Could you check a few things on this model? Use its own coordinates, in mm. A direction names the side the tool comes from. Give positions to 0.01 mm unless a question says otherwise; leave off trailing zeros. Loops run counter-clockwise (first coordinate to the right, second up) from the corner with the lowest first, then second, coordinate; pieces in that order, holes last. Notation, with made-up numbers: (0, 81.5) -> (34, 81.5) arc R28 cw to (34, 110.5) -> close; hole circle Ø4 at (63.25, 44). An arc over 180 degrees is marked (long way). Write item = value, one per line. Start each with the question number.
1) I want a section at A-A (x = -1.25). List the corners of the cut face in (y, z) for me.
2) I want a section at D-D (z = 7.25). List the corners of the cut face in (x, y) for me (3 decimals), and give its area (3 significant figures).
3) I want a section at C-C (z = 0.5). Count the separate pieces of the cut face and the enclosed holes in it, and give its area (3 significant figures).
4) If we mould it in two halves opening along Y, with no side actions, what happens to faces 1 (the face through (-10, -12, 10.9)), 2 (the face through (7.805, 8.803, 9.632)), 3 (the face through (12.93, 12.9, 7.54))? For each: +Y half, -Y half, draft (parallel to the pull), parting line (faces both ways), or undercut.
5) I need wall thicknesses on probe 1 along Y at (x, z) = (-10, 6) (3 decimals); probe 2 along X at (y, z) = (10, 7.5) (3 decimals). Which ranges of each line are inside material? Lowest first, please. Write a range as from..to.
6) On a 3-axis mill with a long thin cutter (end or side, diameter ignored), from which of +Z, -Z, +X, -X, +Y, -Y can I reach the whole of each face in a straight line? I mean faces 4 (the face through (7.824, 8.768, -1.232)), 5 (the face through (12.176, -11.232, 9.632)), 6 (the face through (9.46, -12.44, 4.16)), 7 (the face through (-11, -13.5, 1)). Say none if no direction works.
7) I want a section at B-B (y = 7). List the corners of the cut face in (x, z) for me, and give its area (3 significant figures).
8) I'm going to push flat-ended pins straight in: pin 1 Ø1.5 at (x, z) = (-9.5, 4) entering from +Y; pin 2 Ø4 at (x, y) = (-5, -9.5) entering from +Z; pin 3 Ø13.5 at (x, y) = (4.5, 0) entering from -Z. Where does each tip first touch, or does it pass through?
from build123d import *

# Parameters (mm, degrees)
F1_R      = 1.575
F2_DEPTH  = 1.7
F3_R      = 1.575
F4_DEPTH  = 2.5
F5_R      = 2.5
F5_R_2    = 1.575
F6_DEPTH  = 5
F7_R      = 1.575
F8_DEPTH  = 1.7
F9_R      = 1.575
F10_DEPTH = 2.5


with BuildPart() as f2:
    # F1 (on Top) → F2 (new body)
    with BuildSketch(Plane.XY):
        with BuildLine():
            Line((-10.2, 13.5), (-11.5, 13.5))
            ThreePointArc((-11.5, 13.5), (-12.9142135624, 12.9142135624), (-13.5, 11.5))
            Line((-13.5, 11.5), (-13.5, -11.5))
            ThreePointArc((-13.5, -11.5), (-12.9142135624, -12.9142135624), (-11.5, -13.5))
            Line((-11.5, -13.5), (-10.2, -13.5))
            Line((-10.2, -13.5), (10.2, -13.5))
            Line((10.2, -13.5), (11.5, -13.5))
            ThreePointArc((11.5, -13.5), (12.9142135624, -12.9142135624), (13.5, -11.5))
            Line((13.5, -11.5), (13.5, 11.5))
            ThreePointArc((13.5, 11.5), (12.9142135624, 12.9142135624), (11.5, 13.5))
            Line((11.5, 13.5), (10.2, 13.5))
            Line((10.2, 13.5), (-10.2, 13.5))
        make_face()
        with Locations((-10, -10)):
            Circle(F1_R, mode=Mode.SUBTRACT)
        with Locations((10, -10)):
            Circle(F1_R, mode=Mode.SUBTRACT)
        with Locations((-10, 10)):
            Circle(F1_R, mode=Mode.SUBTRACT)
        with Locations((10, 10)):
            Circle(F1_R, mode=Mode.SUBTRACT)
        with BuildLine():
            Line((-5.5434908481, 18.2035445979), (-10.2, 13.5))
            Line((-10.2, 13.5), (10.2, 13.5))
            Line((10.2, 13.5), (5.5434908481, 18.2035445979))
            ThreePointArc((5.5434908481, 18.2035445979), (5.2178432469, 18.4229151093), (4.832839739, 18.5))
            Line((4.832839739, 18.5), (-4.832839739, 18.5))
            ThreePointArc((-4.832839739, 18.5), (-5.2178432469, 18.4229151093), (-5.5434908481, 18.2035445979))
        make_face()
        with BuildLine():
            Line((10.2, -13.5), (-10.2, -13.5))
            Line((-10.2, -13.5), (-5.5434908481, -18.2035445979))
            ThreePointArc((-5.5434908481, -18.2035445979), (-5.2178432469, -18.4229151093), (-4.832839739, -18.5))
            Line((-4.832839739, -18.5), (4.832839739, -18.5))
            ThreePointArc((4.832839739, -18.5), (5.2178432469, -18.4229151093), (5.5434908481, -18.2035445979))
            Line((5.5434908481, -18.2035445979), (10.2, -13.5))
        make_face()
    extrude(amount=F2_DEPTH)

    # F3 (on face) → F4 (join)
    with BuildSketch(Plane(origin=(0, 0, 0), x_dir=(1, 0, 0), z_dir=(0, 0, -1))):
        Polygon((-11.4020402321, -7.4765863358), (-12.8863604535, -9.952495626), (-11.4843202214, -12.4759092903), (-8.5979597679, -12.5234136642), (-7.1136395465, -10.047504374), (-8.5156797786, -7.5240907097), align=None)
        with Locations((-10, -10)):
            Circle(F3_R, mode=Mode.SUBTRACT)
        Polygon((-12.8863604535, 9.952495626), (-11.4020402321, 7.4765863358), (-8.5156797786, 7.5240907097), (-7.1136395465, 10.047504374), (-8.5979597679, 12.5234136642), (-11.4843202214, 12.4759092903), align=None)
        with Locations((-10, 10)):
            Circle(F3_R, mode=Mode.SUBTRACT)
        Polygon((11.4843202214, -12.4759092903), (12.8863604535, -9.952495626), (11.4020402321, -7.4765863358), (8.5156797786, -7.5240907097), (7.1136395465, -10.047504374), (8.5979597679, -12.5234136642), align=None)
        with Locations((10, -10)):
            Circle(F3_R, mode=Mode.SUBTRACT)
        Polygon((8.5979597679, 12.5234136642), (7.1136395465, 10.047504374), (8.5156797786, 7.5240907097), (11.4020402321, 7.4765863358), (12.8863604535, 9.952495626), (11.4843202214, 12.4759092903), align=None)
        with Locations((10, 10)):
            Circle(F3_R, mode=Mode.SUBTRACT)
    extrude(amount=F4_DEPTH)

    # F5 (on face) → F6 (join)
    with BuildSketch(Plane.XY.offset(1.7)):
        with Locations((-10, 10)):
            Circle(F5_R)
        with Locations((-10, 10)):
            Circle(F5_R_2, mode=Mode.SUBTRACT)
        with Locations((10, 10)):
            Circle(F5_R)
        with Locations((10, 10)):
            Circle(F5_R_2, mode=Mode.SUBTRACT)
        with Locations((10, -10)):
            Circle(F5_R)
        with Locations((10, -10)):
            Circle(F5_R_2, mode=Mode.SUBTRACT)
        with Locations((-10, -10)):
            Circle(F5_R)
        with Locations((-10, -10)):
            Circle(F5_R_2, mode=Mode.SUBTRACT)
    extrude(amount=F6_DEPTH)

    # F7 (on face) → F8 (join)
    with BuildSketch(Plane.XY.offset(6.7)):
        with BuildLine():
            Line((-11.5, -13.5), (11.5, -13.5))
            ThreePointArc((11.5, -13.5), (12.9142135624, -12.9142135624), (13.5, -11.5))
            Line((13.5, -11.5), (13.5, 11.5))
            ThreePointArc((13.5, 11.5), (12.9142135624, 12.9142135624), (11.5, 13.5))
            Line((11.5, 13.5), (-11.5, 13.5))
            ThreePointArc((-11.5, 13.5), (-12.9142135624, 12.9142135624), (-13.5, 11.5))
            Line((-13.5, 11.5), (-13.5, -11.5))
            ThreePointArc((-13.5, -11.5), (-12.9142135624, -12.9142135624), (-11.5, -13.5))
        make_face()
        with Locations((-10, -10)):
            Circle(F7_R, mode=Mode.SUBTRACT)
        with Locations((10, -10)):
            Circle(F7_R, mode=Mode.SUBTRACT)
        with Locations((-10, 10)):
            Circle(F7_R, mode=Mode.SUBTRACT)
        with Locations((10, 10)):
            Circle(F7_R, mode=Mode.SUBTRACT)
    extrude(amount=F8_DEPTH)

    # F9 (on face) → F10 (join)
    with BuildSketch(Plane.XY.offset(8.4)):
        Polygon((-11.4020402321, 7.4765863358), (-8.5156797786, 7.5240907097), (-7.1136395465, 10.047504374), (-8.5979597679, 12.5234136642), (-11.4843202214, 12.4759092903), (-12.8863604535, 9.952495626), align=None)
        with Locations((-10, 10)):
            Circle(F9_R, mode=Mode.SUBTRACT)
        Polygon((12.8863604535, -9.952495626), (11.4020402321, -7.4765863358), (8.5156797786, -7.5240907097), (7.1136395465, -10.047504374), (8.5979597679, -12.5234136642), (11.4843202214, -12.4759092903), align=None)
        with Locations((10, -10)):
            Circle(F9_R, mode=Mode.SUBTRACT)
        Polygon((12.8863604535, 9.952495626), (11.4843202214, 12.4759092903), (8.5979597679, 12.5234136642), (7.1136395465, 10.047504374), (8.5156797786, 7.5240907097), (11.4020402321, 7.4765863358), align=None)
        with Locations((10, 10)):
            Circle(F9_R, mode=Mode.SUBTRACT)
        Polygon((-11.4843202214, -12.4759092903), (-8.5979597679, -12.5234136642), (-7.1136395465, -10.047504374), (-8.5156797786, -7.5240907097), (-11.4020402321, -7.4765863358), (-12.8863604535, -9.952495626), align=None)
        with Locations((-10, -10)):
            Circle(F9_R, mode=Mode.SUBTRACT)
    extrude(amount=F10_DEPTH)


solid = f2.part
Answer list:
q1.outline = (-18.5, 0) -> (18.5, 0) -> (18.5, 1.7) -> (-18.5, 1.7) -> close; (-13.5, 6.7) -> (13.5, 6.7) -> (13.5, 8.4) -> (-13.5, 8.4) -> close
q2.outline = (-13.5, -11.5) arc R2 ccw to (-11.5, -13.5) -> (11.5, -13.5) arc R2 ccw to (13.5, -11.5) -> (13.5, 11.5) arc R2 ccw to (11.5, 13.5) -> (-11.5, 13.5) arc R2 ccw to (-13.5, 11.5) -> close; hole circle Ø3.15 at (-10, -10); hole circle Ø3.15 at (-10, 10); hole circle Ø3.15 at (10, -10); hole circle Ø3.15 at (10, 10)
q2.area = 694 mm^2
q3.separate_pieces = 1
q3.enclosed_holes = 4
q3.area = 849 mm^2
q4.face_1 = draft
q4.face_2 = undercut
q4.face_3 = +Y half
q5.probe_1 = -12.5..-11.575, -8.425..-7.5, 7.5..8.425, 11.575..12.5
q5.probe_2 = -13.5..-11.575, -8.425..8.425, 11.575..13.5
q6.face_4 = -Z
q6.face_5 = +Z, +X, -Y
q6.face_6 = none
q6.face_7 = +Z, -Z, -X, -Y
q7.outline = (-13.5, 0) -> (13.5, 0) -> (13.5, 1.7) -> (-13.5, 1.7) -> close; (-13.5, 6.7) -> (13.5, 6.7) -> (13.5, 8.4) -> (-13.5, 8.4) -> close
q7.area = 91.8 mm^2
q8.pin_1 = 12.5
q8.pin_2 = 8.4
q8.pin_3 = 0
